The model under review builds one solid part; all positions refer to its coordinate system, in mm. Face numbers are marked on the shaded views. A direction names the side the tool comes from. Coordinates: 2 decimals unless noted, no trailing zeros. Write each loop counter-clockwise with the first axis right and the second up, starting at its lowest first coordinate (ties: lowest second). Pieces come first, ordered by that corner, then holes. Notation, with made-up numbers: M 50,43 L 109,43 A21 cw 109,74 Z; hole C -10.75,71.5 d5. An arc over 180 degrees is marked long. Answer as a JSON object with one key per item and string values.
```python
from build123d import *

# Parameters (mm, degrees)
SKETCH_1_R          = 2
EXTRUDE_1_DEPTH     = 5
SKETCH_2_R          = 3
EXTRUDE_2_DEPTH     = 10
EXTRUDE_START       = 4.5
EXTRUDE_3_DEPTH     = 4.5
CUT_EXTRUDE_1_DEPTH = 4.5
CUT_EXTRUDE_START   = -10
SKETCH_7_R          = 2
CUT_EXTRUDE_2_DEPTH = 10
SKETCH_8_R          = 2
CUT_EXTRUDE_3_DEPTH = 10
CUT_EXTRUDE_4_DEPTH = 6
SKETCH_10_W         = 23.139372947
SKETCH_10_H         = 31.36360791
CUT_EXTRUDE_7_DEPTH = 2.8


with BuildPart() as part:
    # 草图1 → 凸台-拉伸1 (new body)
    with BuildSketch(Plane(origin=(0, 0, 0), x_dir=(1, 0, 0), z_dir=(0, 1, 0))):
        with BuildLine():
            Line((0, 10), (100, 10))
            ThreePointArc((100, 10), (110, 0), (100, -10))
            Line((100, -10), (0, -10))
            ThreePointArc((0, -10), (-10, 0), (0, 10))
        make_face()
        with Locations(Location((0, 0, 0), (0, 0, 270))):
            Circle(SKETCH_1_R, mode=Mode.SUBTRACT)
    extrude(amount=EXTRUDE_1_DEPTH)

    # 草图2 → 凸台-拉伸2 (add)
    with BuildSketch(Plane(origin=(0, 5, 0), x_dir=(1, 0, 0), z_dir=(0, 1, 0))):
        with Locations(Location((100, 0, 0), (0, 0, 270))):
            Circle(SKETCH_2_R)
    extrude(amount=EXTRUDE_2_DEPTH)

    # 草图3 → 凸台-拉伸3 (add)
    with BuildSketch(Plane.XZ.offset(EXTRUDE_START)):
        with BuildLine():
            Line((100, 10), (73.40776322, 10))
            Line((73.40776322, 10), (73.40776322, -10))
            Line((73.40776322, -10), (100, -10))
            ThreePointArc((100, -10), (110, 0), (100, 10))
        make_face()
    extrude(amount=-EXTRUDE_3_DEPTH)

    # 草图4 → 切除-拉伸1 (cut)
    with BuildSketch(Plane.XZ.offset(4.5)):
        with BuildLine():
            Line((79.849230428, 2.288593229), (99.690178504, 3.236180981))
            ThreePointArc((99.690178504, 3.236180981), (103.250977807, 0), (99.690178504, -3.236180981))
            Line((99.690178504, -3.236180981), (79.849230428, -2.288593229))
            ThreePointArc((79.849230428, -2.288593229), (77.560637199, 0), (79.849230428, 2.288593229))
        make_face()
    extrude(amount=-CUT_EXTRUDE_1_DEPTH, mode=Mode.SUBTRACT)

    # 草图7 → 切除-拉伸2 (cut)
    with BuildSketch(Plane(origin=(0, 5, 0), x_dir=(1, 0, 0), z_dir=(0, 1, 0)).offset(CUT_EXTRUDE_START)):
        with BuildLine():
            ThreePointArc((58.924703642, -10), (48.924703642, 0), (58.924703642, 10))
            Line((58.924703642, 10), (0, 10))
            ThreePointArc((0, 10), (-10, 0), (0, -10))
            Line((0, -10), (58.924703642, -10))
        make_face()
        Circle(SKETCH_7_R, mode=Mode.SUBTRACT)
    extrude(amount=CUT_EXTRUDE_2_DEPTH, mode=Mode.SUBTRACT)

    # 草图8 → 切除-拉伸3 (cut)
    with BuildSketch(Plane(origin=(0, 5, 0), x_dir=(1, 0, 0), z_dir=(0, 1, 0))):
        with Locations(Location((58.924703642, 0, 0), (0, 0, 270))):
            Circle(SKETCH_8_R)
    extrude(amount=-CUT_EXTRUDE_3_DEPTH, mode=Mode.SUBTRACT)

    # 草图9 → 切除-拉伸4 (cut)
    with BuildSketch(Plane.XZ.offset(4.5)):
        with BuildLine():
            Line((79.849230428, 2.288593229), (99.378953737, 4.81012209))
            ThreePointArc((99.378953737, 4.81012209), (104.850048761, 0), (99.378953737, -4.81012209))
            Line((99.378953737, -4.81012209), (79.849230428, -2.288593229))
            ThreePointArc((79.849230428, -2.288593229), (77.560637199, 0), (79.849230428, 2.288593229))
        make_face()
    extrude(amount=-CUT_EXTRUDE_4_DEPTH, mode=Mode.SUBTRACT)

    # 草图10 → 切除-拉伸7 (cut)
    with BuildSketch(Plane(origin=(0, 15, 0), x_dir=(1, 0, 0), z_dir=(0, 1, 0))):
        with Locations((93.670893517, -8.00991687)):
            Rectangle(SKETCH_10_W, SKETCH_10_H)
    extrude(amount=-CUT_EXTRUDE_7_DEPTH, mode=Mode.SUBTRACT)


solid = part.part
```
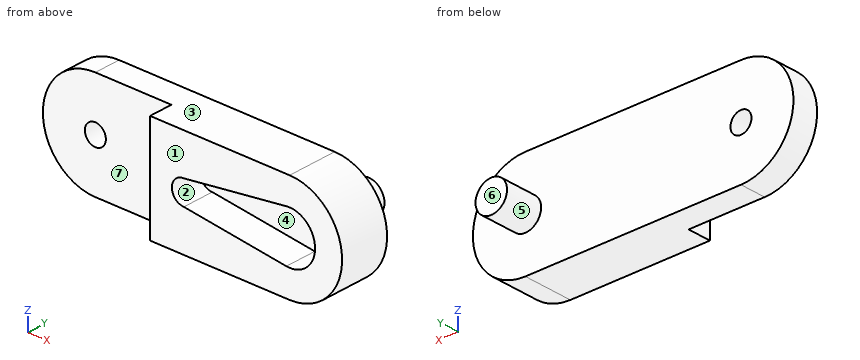
(1) Add section C-C on x = 84.5. Give the boundary of the cut face in (y, z), and give its area (3 significant figures).
Results list:
{"outline": "M -4.5,-10 L 5,-10 L 5,10 L -4.5,10 L -4.5,2.89 L 1.5,2.89 L 1.5,-2.89 L -4.5,-2.89 Z", "area": "155 mm²"}
(2) For the marked faces 4, 5, 6 and 7, list the 3-axis set-ups (+Z, -Z, +X, -X, +Y, -Y) from which the entire face can be reached by the end or side of a thin tool; tool diameter is ignored.
Results list:
{"face 4": "-Y", "face 5": "+Y", "face 6": "+Z, -Z, +X, -X, +Y", "face 7": "+Z, -Z, -X, -Y"}
(3) Add section A-A on z = 0. Give the boundary of the cut face in (x, y), and give its area (3 significant figures).
Results list:
{"outline": "M 48.92,0 L 56.92,0 L 56.92,5 L 48.92,5 Z; M 60.92,0 L 73.41,0 L 73.41,-4.5 L 77.56,-4.5 L 77.56,1.5 L 104.85,1.5 L 104.85,-4.5 L 110,-4.5 L 110,5 L 103,5 L 103,12.2 L 97,12.2 L 97,5 L 60.92,5 Z", "area": "330 mm²"}
(4) Wall thickness on line 1 along X through (y, z) = (1.4, 0); line 2 along Z through (x, y) = (100, -1.2); line 3 along X through (y, z) = (2, 0): over which ranges is each line inside the solid? List them lowest first. Write a range as from..to.
Results list:
{"line 1": "48.92..56.92, 60.92..77.56, 104.85..110", "line 2": "-10..-4.85, 4.85..10", "line 3": "48.92..56.92, 60.92..110"}
(5) Add section D-D on z = -4. Give the boundary of the cut face in (x, y), and give its area (3 significant figures).
Results list:
{"outline": "M 49.76,0 L 73.41,0 L 73.41,-4.5 L 93.1,-4.5 L 93.1,1.5 L 102.74,1.5 L 102.74,-4.5 L 109.17,-4.5 L 109.17,5 L 49.76,5 Z", "area": "400 mm²"}
(6) Draft analysis for pull direction Z (two halves, no side actions). For the marked faces 1, 2 and 3, state which applies: released by +Z, released by -Z, zero draft, split by the parting line, or undercut.
Results list:
{"face 1": "zero draft", "face 2": "undercut", "face 3": "released by +Z"}
(7) For pin 1 Ø5 at (y, z) = (-2, 4.5) entering from -X; pin 2 Ø1 at (x, z) = (59, 5.5) entering from -Y; pin 3 Ø1.5 at (x, y) = (103.5, 8.5) entering from -Z, all flat-tipped, find the tip position at first contact; note any pin that passes through.
Results list:
{"pin 1": "x = 49.39", "pin 2": "y = 0", "pin 3": "z = -1.2"}
(8) Add section B-B on y = -2. Give the boundary of the cut face in (x, z).
Results list:
{"outline": "M 73.41,-10 L 100,-10 A10 ccw 100,10 L 73.41,10 Z; hole M 79.85,-2.29 L 99.38,-4.81 A4.85 ccw long 99.38,4.81 L 79.85,2.29 A2.29 ccw Z"}
